```python
from build123d import *

# Parameters (mm, degrees)
SKETCH2_R           = 60
BOSS_EXTRUDE1_DEPTH = 5
SKETCH3_R           = 8
CUT_EXTRUDE1_DEPTH  = 86
SKETCH4_R           = 10
CUT_EXTRUDE2_DEPTH  = 3
CIRPATTERN1_COUNT   = 6
SKETCH5_R           = 1.5
CUT_EXTRUDE3_DEPTH  = 86
CIRPATTERN2_COUNT   = 6
SKETCH6_W           = 8
SKETCH6_H           = 4
CUT_EXTRUDE4_DEPTH  = 86
FILLET1_R           = 1.5


with BuildPart() as part:
    # Sketch2 → Boss-Extrude1 (new body)
    with BuildSketch(Plane(origin=(0, 0, 0), x_dir=(1, 0, 0), z_dir=(0, 1, 0))):
        with Locations(Location((0, 0, 0), (0, 0, 270))):
            Circle(SKETCH2_R)
    extrude(amount=BOSS_EXTRUDE1_DEPTH)

    # Sketch3 → Cut-Extrude1 (cut, through all)
    with BuildSketch(Plane(origin=(0, 5, 0), x_dir=(1, 0, 0), z_dir=(0, 1, 0))):
        with Locations(Location((0, 0, 0), (0, 0, 270))):
            Circle(SKETCH3_R)
    extrude(amount=-CUT_EXTRUDE1_DEPTH, mode=Mode.SUBTRACT)

    # Sketch4 → Cut-Extrude2 (cut)
    with BuildSketch(Plane(origin=(0, 5, 0), x_dir=(1, 0, 0), z_dir=(0, 1, 0))):
        with Locations(Location((0, 40, 0), (0, 0, 270))):
            Circle(SKETCH4_R)
    cut_extrude2 = extrude(amount=-CUT_EXTRUDE2_DEPTH, mode=Mode.SUBTRACT)

    # CirPattern1: Cut-Extrude2 ×6 about axis
    cirpattern1_axis = Axis((0, 0, 0), (0, 1, 0))
    for i in range(1, CIRPATTERN1_COUNT):
        add(cut_extrude2.rotate(cirpattern1_axis, i * 360 / CIRPATTERN1_COUNT), mode=Mode.SUBTRACT)

    # Sketch5 → Cut-Extrude3 (cut, through all)
    with BuildSketch(Plane(origin=(0, 5, 0), x_dir=(1, 0, 0), z_dir=(0, 1, 0))):
        with Locations(Location((0, 54, 0), (0, 0, 270))):
            Circle(SKETCH5_R)
    cut_extrude3 = extrude(amount=-CUT_EXTRUDE3_DEPTH, mode=Mode.SUBTRACT)

    # CirPattern2: Cut-Extrude3 ×6 about axis
    cirpattern2_axis = Axis((0, 0, 0), (0, 1, 0))
    for i in range(1, CIRPATTERN2_COUNT):
        add(cut_extrude3.rotate(cirpattern2_axis, i * 360 / CIRPATTERN2_COUNT), mode=Mode.SUBTRACT)

    # Sketch6 → Cut-Extrude4 (cut, through all)
    with BuildSketch(Plane(origin=(0, 5, 0), x_dir=(1, 0, 0), z_dir=(0, 1, 0))):
        with Locations((0, 58.067002871)):
            Rectangle(SKETCH6_W, SKETCH6_H)
    extrude(amount=-CUT_EXTRUDE4_DEPTH, mode=Mode.SUBTRACT)

    # Fillet1
    fillet1_edges = [part.edges().sort_by_distance(p)[0] for p in [
        (59.966620262, 0, 2.001113277),
        (-59.966620262, 5, 2.001113277),
    ]]
    fillet(fillet1_edges, radius=FILLET1_R)


solid = part.part
```
CAD build for the part. Positions are in the model's coordinates, mm. A direction names the side the tool comes from. Round coordinates to 2 decimals unless told otherwise and drop trailing zeros. Use a Markdown table: item, result. Add a question column.
(1) Drill centre lines: line 1 (Z direction, x = -36, y = 3.5); line 2 (X direction, y = 2.7, z = -23.5); line 3 (X direction, y = 3, z = -27). Where is each one in solid material? Low to high.
(2) Which spindle directions (+Z, -Z, +X, -X, +Y, -Y) get a long thin tool onto all of the face, cutting with end or side? Do faces 4 (the face through (-12, 0, -1)), 5 (the face through (0, 2, -40)). Say none if no direction does.
(3) Flat gauge pins, fed straight in: pin 1 (16 mm diameter, centred on x = -34.64, z = -20, fed in from +Y); pin 2 (3 mm diameter, centred on x = -9.5, y = 3, fed in from +Z); pin 3 (3 mm diameter, centred on y = 2.5, z = -36, fed in from +X). Where does each tip first touch, or does it go through?
(4) Pull direction Z, two halves, no side cores. Call faces 1 (the face through (-12, 5, -1)), 2 (the face through (-35, 2, 20)), 3 (the face through (0, 3, -56.067)): +Z half, -Z half, draft (parallel to the pull), parting line (faces both ways), or undercut.
Geometry says:
| question | item | result |
|---|---|---|
| 1 | line 1 | z = -48 to -29.91, -10.09 to 10.09, 29.91 to 48 |
| 1 | line 2 | x = -55.21 to -44.01, -25.27 to 25.27, 44.01 to 55.21 |
| 1 | line 3 | x = -53.58 to -48.27, -45.27 to -41.78, -27.5 to 27.5, 41.78 to 45.27, 48.27 to 53.58 |
| 2 | face 4 | +Z, -Z, +X, -X, -Y |
| 2 | face 5 | +Y |
| 3 | pin 1 | stops at y = 2 |
| 3 | pin 2 | stops at z = 59.46 |
| 3 | pin 3 | stops at x = 49.09 |
| 4 | face 1 | draft |
| 4 | face 2 | undercut |
| 4 | face 3 | -Z half |
